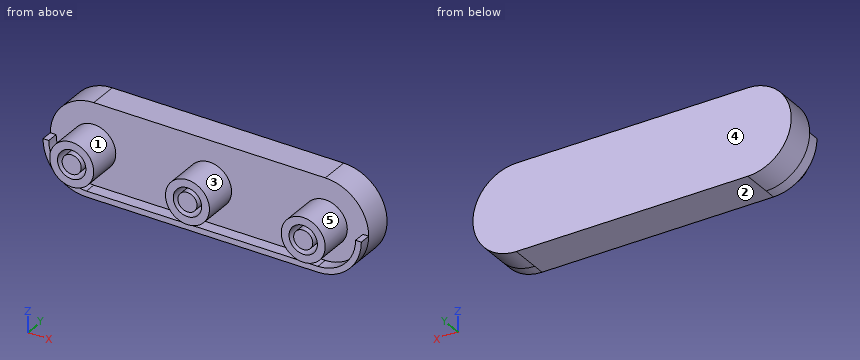
```python
from build123d import *

# Parameters (mm, degrees)
SKETCH1_R        = 2.0955
PLUGS_DEPTH      = 7.62
SKETCH1_R_2      = 4.826
SKETCH1_R_3      = 3.1115
PLUGS_2_DEPTH    = 7.62
PLUGS_3_DEPTH    = 7.62
PLUGS_4_DEPTH    = 7.62
PLUGS_5_DEPTH    = 7.62
PLUGS_6_DEPTH    = 7.62
BACK_PLATE_DEPTH = 6.35
RAIN_GUARD_DEPTH = 2.54


with BuildPart() as part:
    # Sketch1 → Plugs (new body)
    with BuildSketch(Plane(origin=(0, 0, 0), x_dir=(1, 0, 0), z_dir=(0, 1, 0))):
        with Locations((-25.4, 0)):
            Circle(SKETCH1_R)
    extrude(amount=PLUGS_DEPTH)



with BuildPart() as body_2:
    # Sketch1 → Plugs 2 (new body)
    with BuildSketch(Plane(origin=(0, 0, 0), x_dir=(1, 0, 0), z_dir=(0, 1, 0))):
        with Locations((-25.4, 0)):
            Circle(SKETCH1_R_2)
        with Locations((-25.4, 0)):
            Circle(SKETCH1_R_3, mode=Mode.SUBTRACT)
    extrude(amount=PLUGS_2_DEPTH)


with BuildPart() as body_3:
    # Sketch1 → Plugs 3 (new body)
    with BuildSketch(Plane(origin=(0, 0, 0), x_dir=(1, 0, 0), z_dir=(0, 1, 0))):
        Circle(SKETCH1_R)
    extrude(amount=PLUGS_3_DEPTH)


with BuildPart() as body_4:
    # Sketch1 → Plugs 4 (new body)
    with BuildSketch(Plane(origin=(0, 0, 0), x_dir=(1, 0, 0), z_dir=(0, 1, 0))):
        Circle(SKETCH1_R_2)
        Circle(SKETCH1_R_3, mode=Mode.SUBTRACT)
    extrude(amount=PLUGS_4_DEPTH)


with BuildPart() as body_5:
    # Sketch1 → Plugs 5 (new body)
    with BuildSketch(Plane(origin=(0, 0, 0), x_dir=(1, 0, 0), z_dir=(0, 1, 0))):
        with Locations((25.4, 0)):
            Circle(SKETCH1_R)
    extrude(amount=PLUGS_5_DEPTH)


with BuildPart() as body_6:
    # Sketch1 → Plugs 6 (new body)
    with BuildSketch(Plane(origin=(0, 0, 0), x_dir=(1, 0, 0), z_dir=(0, 1, 0))):
        with Locations((25.4, 0)):
            Circle(SKETCH1_R_2)
        with Locations((25.4, 0)):
            Circle(SKETCH1_R_3, mode=Mode.SUBTRACT)
    extrude(amount=PLUGS_6_DEPTH)


with BuildPart() as part_1:
    add(part.part)

    add(body_2.part)  # Back Plate merges body 2

    add(body_3.part)  # Back Plate merges body 3

    add(body_4.part)  # Back Plate merges body 4

    add(body_5.part)  # Back Plate merges body 5

    add(body_6.part)  # Back Plate merges body 6
    # Sketch2 → Back Plate (add)
    with BuildSketch(Plane(origin=(0, 7.62, 0), x_dir=(1, 0, 0), z_dir=(0, 1, 0))):
        with BuildLine():
            Line((-25.4, 9.525), (25.4, 9.525))
            ThreePointArc((25.4, 9.525), (34.925, 0), (25.4, -9.525))
            Line((25.4, -9.525), (-25.4, -9.525))
            ThreePointArc((-25.4, -9.525), (-34.925, 0), (-25.4, 9.525))
        make_face()
    extrude(amount=BACK_PLATE_DEPTH)

    # Sketch3 → Rain Guard (add)
    with BuildSketch(Plane.XZ.offset(-7.62)):
        with BuildLine():
            Line((25.4, -9.525), (-25.4, -9.525))
            ThreePointArc((-25.4, -9.525), (-32.135192091, -6.735192091), (-34.925, 0))
            Line((-34.925, 0), (-33.655, 0))
            ThreePointArc((-33.655, 0), (-31.237166479, -5.837166479), (-25.4, -8.255))
            Line((-25.4, -8.255), (25.4, -8.255))
            ThreePointArc((25.4, -8.255), (31.237166479, -5.837166479), (33.655, 0))
            Line((33.655, 0), (34.925, 0))
            ThreePointArc((34.925, 0), (32.135192091, -6.735192091), (25.4, -9.525))
        make_face()
    extrude(amount=RAIN_GUARD_DEPTH)


solid = part_1.part
```
For this review, take the finished solid that the model builds, in its own axes (mm). Face numbers are marked on the shaded views. A direction names the side the tool comes from. Coordinates: 2 decimals unless noted, no trailing zeros. Write each loop counter-clockwise with the first axis right and the second up, starting at its lowest first coordinate (ties: lowest second). Pieces come first, ordered by that corner, then holes.
(1) Add section D-D on z = -5.75. Give the boundary of the cut face in (x, y), then the cut area to 3 significant figures.
(2) Add section B-B on x = 0. Give the boundary of the cut face in (y, z) (1 decimal), then the cut area to 3 significant figures.
(3) Wall thickness on probe 1 along Z at (x, y) = (-25.4, 1.5); probe 2 along Y at (x, z) = (-16.5, 8.25); probe 3 along Z at (x, y) = (17, 7.25) (3 decimals): over which ranges is each line inside the solid? List them lowest first.
(4) For pin 1 Ø1.5 at (x, z) = (6.5, 4.5) entering from -Y; pin 2 Ø1 at (y, z) = (6, -3.5) entering from +X; pin 3 Ø4 at (x, y) = (8, 2.5) entering from -Z; pin 4 Ø0.8 at (x, y) = (-0.5, 6.5) entering from +Z, all flat-tipped, find the tip position at first contact; note any pin that passes through.
(5) Add section C-C on y = 8.5. Give the boundary of the cut face in (x, z) (3 decimals).
(6) Add section A-A on y = 2. Count the separate pieces of the cut face and the enclosed holes in it, then the cut area to 3 significant figures.
(7) Tool access review of the marked faces 1 and 2: name each direction out of +Z, -Z, +X, -X, +Y, -Y from which nothing blocks a thin tool from reaching the whole face with its end or side.
(8) The part is to be moulded in two halves that separate along X. For the marked faces 3, 4 and 5, say which applies: +X half, -X half, draft (parallel to the pull), parting line (faces both ways), or undercut.
Answer sheet:
1. outline: (-32.99, 5.08) - (-31.32, 5.08) - (-31.32, 7.62) - (31.32, 7.62) - (31.32, 5.08) - (32.99, 5.08) - (32.99, 13.97) - (-32.99, 13.97) - close
1. area: 428 mm2
2. outline: (0, -4.8) - (7.6, -4.8) - (7.6, -8.3) - (5.1, -8.3) - (5.1, -9.5) - (14, -9.5) - (14, 9.5) - (7.6, 9.5) - (7.6, 4.8) - (0, 4.8) - (0, 3.1) - (7.6, 3.1) - (7.6, 2.1) - (0, 2.1) - (0, -2.1) - (7.6, -2.1) - (7.6, -3.1) - (0, -3.1) - close
2. area: 182 mm2
3. probe 1: z = -4.83 to -3.11, -2.1 to 2.1, 3.11 to 4.83
3. probe 2: y = 7.62 to 13.97
3. probe 3: z = -9.525 to -8.255
4. pin 1: stops at y = 7.62
4. pin 2: stops at x = 34.44
4. pin 3: passes through
4. pin 4: stops at z = 4.82
5. outline: (-25.4, -9.525) - (25.4, -9.525) arc R9.525 ccw to (25.4, 9.525) - (-25.4, 9.525) arc R9.525 ccw to start
6. separate pieces: 6
6. enclosed holes: 3
6. area: 170 mm2
7. face 1: -Y
7. face 2: -Z, +X, -X, +Y, -Y
8. face 3: undercut
8. face 4: draft
8. face 5: undercut
